```python
from build123d import *

# Parameters (mm, degrees)
SKETCH1_R           = 35
SKETCH1_R_2         = 31
BOSS_EXTRUDE1_DEPTH = 36
BOSS_EXTRUDE3_START = -27
BOSS_EXTRUDE3_DEPTH = 27
SKETCH7_W           = 13.353088805
SKETCH7_H           = 12.6
BOSS_EXTRUDE4_DEPTH = 20
SKETCH8_W           = 17
SKETCH8_H           = 12.6
BOSS_EXTRUDE5_DEPTH = 5
BOSS_EXTRUDE6_DEPTH = 6.5
BOSS_EXTRUDE2_START = -35
BOSS_EXTRUDE2_DEPTH = 35


# Read off the part's stored shape, not the designer's step: Boss-Extrude6
with BuildPart() as part:
    # Sketch1 → Boss-Extrude1 (new body)
    with BuildSketch(Plane.XY):
        Circle(SKETCH1_R)
        Circle(SKETCH1_R_2, mode=Mode.SUBTRACT)
    extrude(amount=BOSS_EXTRUDE1_DEPTH)

    # Sketch5 → Boss-Extrude3 (add)
    with BuildSketch(Plane.XY.offset(36).offset(BOSS_EXTRUDE3_START)):
        with BuildLine():
            Line((0, 6.3), (0, 9.3))
            Line((0, 9.3), (-29.572115244, 9.3))
            ThreePointArc((-29.572115244, 9.3), (-30.000125334, 7.809768238), (-30.353088805, 6.3))
            Line((-30.353088805, 6.3), (0, 6.3))
        make_face()
        with BuildLine():
            ThreePointArc((-30.353088805, -6.3), (-30.000125334, -7.809768238), (-29.572115244, -9.3))
            Line((-29.572115244, -9.3), (0, -9.3))
            Line((0, -9.3), (0, -6.3))
            Line((0, -6.3), (-30.353088805, -6.3))
        make_face()
    extrude(amount=BOSS_EXTRUDE3_DEPTH)

    # Sketch7 → Boss-Extrude4 (add)
    with BuildSketch(Plane.XY.offset(36)):
        with Locations((-23.676544402, 0)):
            Rectangle(SKETCH7_W, SKETCH7_H)
    extrude(amount=-BOSS_EXTRUDE4_DEPTH)

    # Sketch8 → Boss-Extrude5 (add)
    with BuildSketch(Plane.XY.offset(36)):
        with Locations((-8.5, 0)):
            Rectangle(SKETCH8_W, SKETCH8_H)
    extrude(amount=-BOSS_EXTRUDE5_DEPTH)

    # Boss-Extrude6 outline → Boss-Extrude6 (add)
    with BuildSketch(Plane(origin=(0, 0, 0), x_dir=(0, 0, -1), z_dir=(1, 0, 0))):
        Polygon((-31, 6.3), (-9, 6.3), (-9, 9.3), (-36, 9.3), (-36, -9.3), (-9, -9.3), (-9, -6.3), (-31, -6.3), align=None)
    extrude(amount=BOSS_EXTRUDE6_DEPTH)

    # Sketch2 → Boss-Extrude2 (add)
    with BuildSketch(Plane.XY.offset(36).offset(BOSS_EXTRUDE2_START)):
        with BuildLine():
            Line((0, -6.3), (-30.353088805, -6.3))
            ThreePointArc((-30.353088805, -6.3), (-30.000125334, -7.809768238), (-29.572115244, -9.3))
            Line((-29.572115244, -9.3), (0, -9.3))
            Line((0, -9.3), (0, -6.3))
        make_face()
        with BuildLine():
            Line((-30.353088805, 6.3), (0, 6.3))
            Line((0, 6.3), (0, 9.3))
            Line((0, 9.3), (-29.572115244, 9.3))
            ThreePointArc((-29.572115244, 9.3), (-30.000125334, 7.809768238), (-30.353088805, 6.3))
        make_face()
    extrude(amount=BOSS_EXTRUDE2_DEPTH)


solid = part.part
```
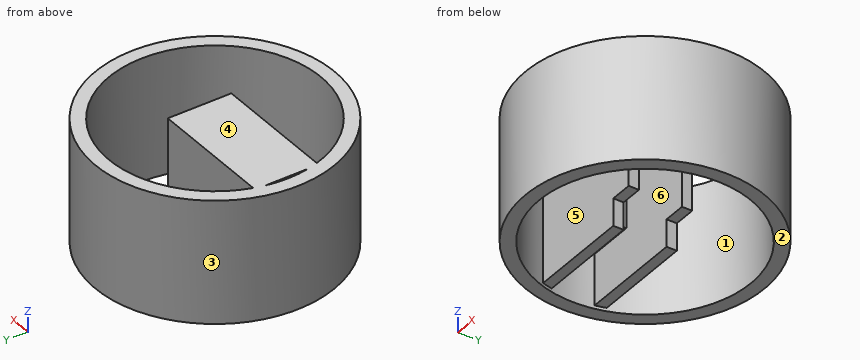
Geometry check sheet. Reference: the model listing, model coordinates, mm. Face numbers are marked on the shaded views. A direction names the side the tool comes from. Coordinates: 2 decimals unless noted, no trailing zeros. Write each loop counter-clockwise with the first axis right and the second up, starting at its lowest first coordinate (ties: lowest second). Pieces come first, ordered by that corner, then holes. Notation, with made-up numbers: M 66.25,19 L 86.25,19 A32 cw 86.25,48 Z; hole C 23,-38.75 d2. An arc over 180 degrees is marked long. One line per item, written item: value. Start each with the question number.
(1) Sectioned sample at B-B, the plane y = 0. Enter the section's corners in (x, z).
(2) Sectioned sample at C-C, the plane x = -10.5. Enter the section's corners in (y, z), and give its area (3 significant figures).
(3) Scan lines: line 1 along Y through (x, z) = (0, 11); line 2 along Y through (x, z) = (5, 10.5); line 3 along X through (y, z) = (26, 28.5). Record each from-to range of solid material in increasing order. Write a range as [from, to].
(4) Depth check by flat-ended pin: pin 1 (1.5 mm diameter, centred on y = -13.5, z = 9, fed in from +X); pin 2 (14 mm diameter, centred on x = -25, y = -0.5, fed in from -Z); pin 3 (1.5 mm diameter, centred on x = 3.5, y = -8, fed in from -Z); pin 4 (5 mm diameter, centred on x = -13, z = 27, fed in from +Y). Enter the tip coordinate at first touch or a pass-through.
(5) Sectioned sample at D-D, the plane y = -20. Enter the section's corners in (x, z), and give its area (3 significant figures).
(6) Sectioned sample at A-A, the plane z = 28. Enter the section's corners in (x, y).
(7) Tool access check on the marked faces 4, 5 and 6. Record the directions out of +Z, -Z, +X, -X, +Y, -Y that give a thin tool (end or side, any length) a straight path to the whole face; none if there is none.
(8) Release check for a two-part mould opening along X. For the marked faces 1, 2 and 3 record: released by +X, released by -X, zero draft, split by the parting line, or undercut.
Filled sheet:
1. outline: M -35,0 L -31,0 L -31,36 L -35,36 Z; M -30.35,16 L -17,16 L -17,31 L 6.5,31 L 6.5,36 L -30.35,36 Z; M 31,0 L 35,0 L 35,36 L 31,36 Z
2. outline: M -33.39,0 L -29.17,0 L -29.17,36 L -33.39,36 Z; M -9.3,1 L -6.3,1 L -6.3,31 L 6.3,31 L 6.3,1 L 9.3,1 L 9.3,36 L -9.3,36 Z; M 29.17,0 L 33.39,0 L 33.39,36 L 29.17,36 Z
2. area: 577 mm²
3. line 1: [-35, -31], [-9.3, -6.3], [6.3, 9.3], [31, 35]
3. line 2: [-34.64, -30.59], [-9.3, -6.3], [6.3, 9.3], [30.59, 34.64]
3. line 3: [-23.43, -16.88], [16.88, 23.43]
4. pin 1: x = 32.6
4. pin 2: z = 0
4. pin 3: z = 9
4. pin 4: y = 33.39
5. outline: M -28.72,0 L -23.69,0 L -23.69,36 L -28.72,36 Z; M 23.69,0 L 28.72,0 L 28.72,36 L 23.69,36 Z
5. area: 363 mm²
6. outline: C 0,0 d70; hole M -30.35,-6.3 L -30.35,6.3 A31 ccw Z; hole M -29.57,-9.3 A31 ccw long -29.57,9.3 L 6.5,9.3 L 6.5,6.3 L -17,6.3 L -17,-6.3 L 6.5,-6.3 L 6.5,-9.3 Z
7. face 4: +Z, +X, -X, +Y, -Y
7. face 5: +Z, -Z
7. face 6: -Z
8. face 1: undercut
8. face 2: zero draft
8. face 3: split by the parting line
